Can you work these out from the model? Positions are in its coordinate system, mm. Face numbers are marked on the shaded views. A direction names the side the tool comes from. Coordinates: 2 decimals unless noted, no trailing zeros. Order: outer loops, then holes, each group sorted by start corner. A loop starts at its lowest first (then second) coordinate and runs counter-clockwise, first axis right, second up. Notation, with made-up numbers: (80.5, 45.25) -> (91.5, 45.25) arc R17 ccw to (91.5, 74.25) -> close; hole circle Ø5 at (84, 56). An arc over 180 degrees is marked (long way). Answer in a Markdown table with one row per item.
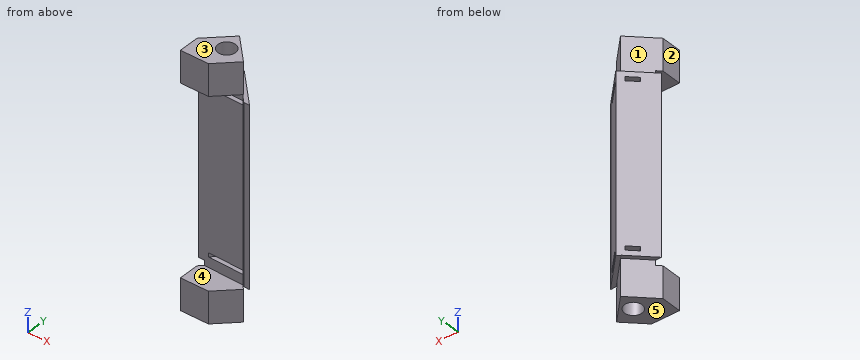
```python
from build123d import *

# Parameters (mm, degrees)
BOSS_EXTRU_1_DEPTH       = 61.5
D_GAGEMENT_M41_D         = 4.3
D_GAGEMENT_M41_DEPTH     = 6
D_GAGEMENT_M41_TIP       = 1.291850331
D_GAGEMENT_M42_D         = 4.3
D_GAGEMENT_M42_DEPTH     = 6
D_GAGEMENT_M42_TIP       = 1.291850331
ESQUISSE9_W              = 1
ESQUISSE9_H              = 6.5
ENL_V_MAT_EXTRU_2_DEPTH  = 66.352343655
ESQUISSE11_W             = 3
ESQUISSE11_H             = 1
ENL_V_MAT_EXTRU_3_DEPTH  = 1
ENL_V_MAT_EXTRU_4_DEPTH  = 23
ENL_V_MAT_EXTRU_7_DEPTH  = 23
ESQUISSE16_W             = 8.145455673
ESQUISSE16_H             = 43.5
ESQUISSE16_W_2           = 3
ESQUISSE16_H_2           = 1
BOSS_EXTRU_2_DEPTH       = 1
ESQUISSE17_W             = 43.576204057
ESQUISSE17_H             = 9.375689411
ESQUISSE17_W_2           = 1
ESQUISSE17_H_2           = 6.5
BOSS_EXTRU_3_DEPTH       = 1
ESQUISSE18_W             = 16.892190225
ESQUISSE18_H             = 46
ENL_V_MAT_EXTRU_8_DEPTH  = 1
BOSS_EXTRU_4_START       = -43.576204
BOSS_EXTRU_4_DEPTH       = 43.576204
ESQUISSE23_W             = 1
ESQUISSE23_H             = 6.5
ENL_V_MAT_EXTRU_11_DEPTH = 66.811115965


with BuildPart() as part:
    # Esquisse1 → Boss.-Extru.1 (new body)
    with BuildSketch(Plane.XY):
        Polygon((-29.2538383, -8.878195219), (-29.2538383, -3.878764136), (-23.419589724, 1.805423729), (-17.574736592, -4.193731626), (-22.3828685, -8.878195219), align=None)
    extrude(amount=BOSS_EXTRU_1_DEPTH)

    # Dégagement M41
    with Locations(Plane.XY.offset(61.5)):
        with Locations((-22.7538383, -2.878195219)):
            Hole(D_GAGEMENT_M41_D / 2, depth=D_GAGEMENT_M41_DEPTH)
            with Locations((0, 0, -(D_GAGEMENT_M41_DEPTH + D_GAGEMENT_M41_TIP / 2))):  # 118° drill point
                Cone(0, D_GAGEMENT_M41_D / 2, D_GAGEMENT_M41_TIP, mode=Mode.SUBTRACT)

    # Dégagement M42
    with Locations(Plane(origin=(0, 0, 0), x_dir=(-1, 0, 0), z_dir=(0, 0, -1))):
        with Locations((22.7538383, -2.878195219)):
            Hole(D_GAGEMENT_M42_D / 2, depth=D_GAGEMENT_M42_DEPTH)
            with Locations((0, 0, -(D_GAGEMENT_M42_DEPTH + D_GAGEMENT_M42_TIP / 2))):  # 118° drill point
                Cone(0, D_GAGEMENT_M42_D / 2, D_GAGEMENT_M42_TIP, mode=Mode.SUBTRACT)

    # Esquisse9 → Enlèv. mat.-Extru.2 (cut, through all)
    with BuildSketch(Plane(origin=(-11.112445005, -10.826625609, 0), x_dir=(0, 0, -1), z_dir=(0.7162580965216612, 0.6978354671175484, 0))):
        with Locations((-50.75, 13.636169698)):
            Rectangle(ESQUISSE9_W, ESQUISSE9_H)
        with Locations((-10.75, 13.636169698)):
            Rectangle(ESQUISSE9_W, ESQUISSE9_H)
    extrude(amount=-ENL_V_MAT_EXTRU_2_DEPTH, mode=Mode.SUBTRACT)

    # Esquisse11 → Enlèv. mat.-Extru.3 (cut)
    with BuildSketch(Plane(origin=(-12.30714472, 12.632049338, 0), x_dir=(0.7162580965216613, 0.6978354671175482, 0), z_dir=(-0.6978354671175482, 0.7162580965216613, 0))):
        with Locations((-17.764582046, -50.75)):
            Rectangle(ESQUISSE11_W, ESQUISSE11_H)
        with Locations((-17.764582046, -10.75)):
            Rectangle(ESQUISSE11_W, ESQUISSE11_H)
    extrude(amount=-ENL_V_MAT_EXTRU_3_DEPTH, mode=Mode.SUBTRACT)

    # Esquisse14 → Enlèv. mat.-Extru.4 (cut)
    with BuildSketch(Plane(origin=(0, 0, 30.75), x_dir=(-1, 0, 0), z_dir=(0, 0, -1))):
        Polygon((22.3828685, -8.878195219), (29.2538383, -3.878764136), (29.2538383, -8.878195219), align=None)
    enl_v_mat_extru_4 = extrude(amount=-ENL_V_MAT_EXTRU_4_DEPTH, mode=Mode.SUBTRACT)

    # Esquisse15 → Enlèv. mat.-Extru.7 (cut)
    with BuildSketch(Plane(origin=(0, 0, 30.75), x_dir=(-1, 0, 0), z_dir=(0, 0, -1))):
        Polygon((17.574736592, -4.193731626), (22.3828685, -8.878195219), (29.2538383, -3.878764136), align=None)
    enl_v_mat_extru_7 = extrude(amount=-ENL_V_MAT_EXTRU_7_DEPTH, mode=Mode.SUBTRACT)

    # Symétrie2: Enlèv. mat.-Extru.4, Enlèv. mat.-Extru.7 across plane
    add(enl_v_mat_extru_4.mirror(Plane(origin=(0, 0, 30.75), x_dir=(1, 0, 0), z_dir=(0, 0, -1))), mode=Mode.SUBTRACT)
    add(enl_v_mat_extru_7.mirror(Plane(origin=(0, 0, 30.75), x_dir=(1, 0, 0), z_dir=(0, 0, -1))), mode=Mode.SUBTRACT)

    # Esquisse16 → Boss.-Extru.2 (add)
    with BuildSketch(Plane(origin=(-12.30714472, 12.632049338, 0), x_dir=(0.7162580965216613, 0.6978354671175481, 0), z_dir=(-0.6978354671175481, 0.7162580965216613, 0))):
        with Locations((-19.587309883, -30.75)):
            Rectangle(ESQUISSE16_W, ESQUISSE16_H)
        with Locations((-17.764582046, -10.75)):
            Rectangle(ESQUISSE16_W_2, ESQUISSE16_H_2, mode=Mode.SUBTRACT)
        with Locations((-17.764582046, -50.75)):
            Rectangle(ESQUISSE16_W_2, ESQUISSE16_H_2, mode=Mode.SUBTRACT)
    extrude(amount=BOSS_EXTRU_2_DEPTH)

    # Esquisse17 → Boss.-Extru.3 (add)
    with BuildSketch(Plane(origin=(-11.112445005, -10.826625609, 0), x_dir=(0, 0, -1), z_dir=(0.7162580965216608, 0.6978354671175485, 0))):
        with Locations((-30.711897972, 13.948324992)):
            Rectangle(ESQUISSE17_W, ESQUISSE17_H)
        with Locations((-50.75, 13.636169698)):
            Rectangle(ESQUISSE17_W_2, ESQUISSE17_H_2, mode=Mode.SUBTRACT)
        with Locations((-10.75, 13.636169698)):
            Rectangle(ESQUISSE17_W_2, ESQUISSE17_H_2, mode=Mode.SUBTRACT)
    extrude(amount=BOSS_EXTRU_3_DEPTH)

    # Esquisse18 → Enlèv. mat.-Extru.8 (cut)
    with BuildSketch(Plane(origin=(-0.12578911, -4.664303021, 0), x_dir=(-0.9996365490865532, 0.026958667072524062, 0), z_dir=(-0.026958667072524065, -0.9996365490865533, 0))):
        with Locations((22.669999121, -30.75)):
            Rectangle(ESQUISSE18_W, ESQUISSE18_H)
    extrude(amount=-ENL_V_MAT_EXTRU_8_DEPTH, mode=Mode.SUBTRACT)

    # Esquisse21 → Boss.-Extru.4 (add)
    with BuildSketch(Plane.XY.offset(52.5).offset(BOSS_EXTRU_4_START)):
        Polygon((-17.141851408, -3.205042293), (-15.591482071, -4.796340876), (-17.025300163, -4.757672998), (-18.575669499, -3.166374415), align=None)
    extrude(amount=BOSS_EXTRU_4_DEPTH)

    # Esquisse23 → Enlèv. mat.-Extru.11 (cut, through all)
    with BuildSketch(Plane(origin=(-10.396186908, -10.128790142, 0), x_dir=(0, 0, -1), z_dir=(0.7162580965216607, 0.6978354671175486, 0))):
        with Locations((-50.75, 13.636169698)):
            Rectangle(ESQUISSE23_W, ESQUISSE23_H)
        with Locations((-10.75, 13.636169698)):
            Rectangle(ESQUISSE23_W, ESQUISSE23_H)
    extrude(amount=-ENL_V_MAT_EXTRU_11_DEPTH, mode=Mode.SUBTRACT)


solid = part.part
```
(1) Will these pins go through, and if not, where does the flat tip stop? pin 1 Ø6 at (y, z) = (-7.5, 40) entering from -X; pin 2 Ø4 at (y, z) = (-6.5, 56) entering from -X; pin 3 Ø4 at (x, y) = (-19.5, 1) entering from -Z.
Response values:
| item | result |
|---|---|
| pin 1 | x = -17.28 |
| pin 2 | x = -29.25 |
| pin 3 | z = 8.92 |
(2) We'd pull the mould along Z, two halves only. Please class the marked faces 3, 4 and 5: +Z half, -Z half, draft (parallel to the pull), parting line (faces both ways), or undercut.
Response values:
| item | result |
|---|---|
| face 3 | +Z half |
| face 4 | undercut |
| face 5 | -Z half |
(3) I need wall thicknesses on line 1 (Z direction, x = -23, y = 0.75); line 2 (Z direction, x = -22.25, y = -6); line 3 (Z direction, x = -24.5, y = -2). Which ranges of each line are inside material? Lowest first, please. Write a range as [from, to].
Response values:
| item | result |
|---|---|
| line 1 | [0, 10.25], [11.25, 50.25], [51.25, 61.5] |
| line 2 | [0, 7.75], [53.75, 61.5] |
| line 3 | [6.12, 10.25], [11.25, 50.25], [51.25, 55.38] |
(4) On a 3-axis mill with a long thin cutter (end or side, diameter ignored), from which of +Z, -Z, +X, -X, +Y, -Y can I reach the whole of each face in a straight line? I mean the marked faces 1 and 2. Say none if no direction works.
Response values:
| item | result |
|---|---|
| face 1 | +Z, -X, +Y |
| face 2 | +Z, -Z, -X, +Y, -Y |
(5) Suppose I cut it at B-B (z = 32). Please give me the cut outline in (x, y).
Response values:
| item | result |
|---|---|
| outline | (-29.65, -2.87) -> (-18.58, -3.17) -> (-17.03, -4.76) -> (-15.59, -4.8) -> (-23.4, 3.22) -> close |
(6) Suppose I cut it at C-C (x = -16.25). Please give me the cut outline in (y, z).
Response values:
| item | result |
|---|---|
| outline | (-4.78, 8.92) -> (-4.12, 8.92) -> (-4.12, 52.5) -> (-4.78, 52.5) -> close |
(7) Suppose I cut it at A-A (y = -7). Please give me the cut outline in (x, z).
Response values:
| item | result |
|---|---|
| outline | (-29.25, 0) -> (-20.46, 0) -> (-20.46, 7.75) -> (-29.25, 7.75) -> close; (-29.25, 53.75) -> (-20.46, 53.75) -> (-20.46, 61.5) -> (-29.25, 61.5) -> close |
